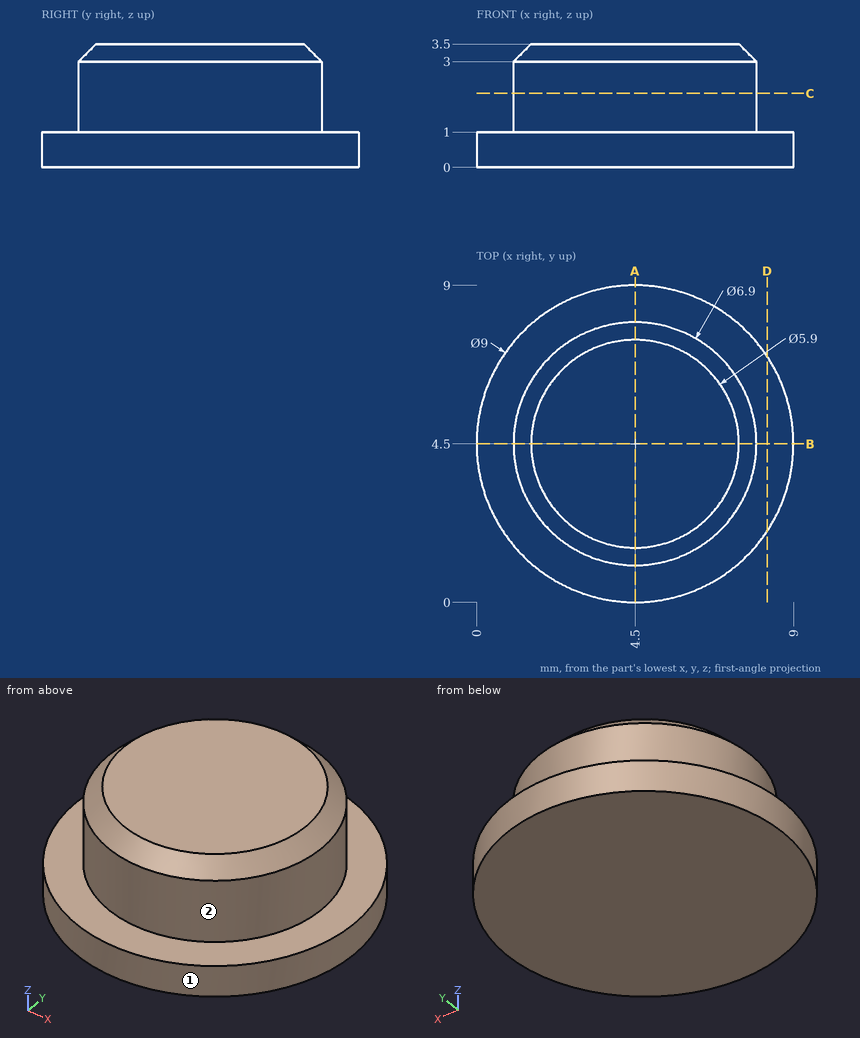
Can you work these out from the drawing? Everything is in mm from the part's minimum corner. A direction names the side the tool comes from. Give positions to 0.01 mm unless a question says otherwise; leave off trailing zeros. Loops run counter-clockwise (first coordinate to the right, second up) from the corner with the lowest first, then second, coordinate; pieces in that order, holes last. Notation, with made-up numbers: (-38.75, -6) -> (1.25, -6) arc R4 cw to (1.25, 0) -> close; hole circle Ø6 at (-8, -12.5). An arc over 180 degrees is marked (long way). Return JSON: item names as keys, results as strings.
Q1. I want a section at C-C, the plane z = 2.1. List the corners of the cut face in (x, y) for me, then the cut area to 3 significant figures.
Checks:
{"outline": "circle Ø6.9 at (4.5, 4.5)", "area": "37.4 mm2"}
Q2. I want a section at D-D, the plane x = 8.25. List the corners of the cut face in (y, z) for me.
Checks:
{"outline": "(2.01, 0) -> (6.99, 0) -> (6.99, 1) -> (2.01, 1) -> close"}
Q3. I need wall thicknesses on probe 1 along Z at (x, y) = (1.75, 7.5); probe 2 along X at (y, z) = (6.25, 0.35); probe 3 along X at (y, z) = (5.75, 0.45). Which ranges of each line are inside material? Lowest first, please.
Checks:
{"probe 1": "z = 0 to 1", "probe 2": "x = 0.35 to 8.65", "probe 3": "x = 0.18 to 8.82"}
Q4. On a 3-axis mill with a long thin cutter (end or side, diameter ignored), from which of +Z, -Z, +X, -X, +Y, -Y can I reach the whole of each face in a straight line? I mean the marked faces 1 and 2. Say none if no direction works.
Checks:
{"face 1": "+Z, -Z", "face 2": "+Z"}
Q5. I want a section at A-A, the plane x = 4.5. List the corners of the cut face in (y, z) for me.
Checks:
{"outline": "(0, 0) -> (9, 0) -> (9, 1) -> (7.95, 1) -> (7.95, 3) -> (7.45, 3.5) -> (1.55, 3.5) -> (1.05, 3) -> (1.05, 1) -> (0, 1) -> close"}
Q6. For pin 1 Ø1.5 at (x, z) = (1.5, 1.5) entering from -Y; pin 2 Ø1.5 at (y, z) = (4, 1.5) entering from +X; pin 3 Ø1.5 at (y, z) = (4, 3) entering from -X; pin 4 Ø1.5 at (y, z) = (1.5, 2.5) entering from -X, each with a flat end and sliding along its axis, tell me the tip position at first contact or that it passes through.
Checks:
{"pin 1": "stops at y = 0.72", "pin 2": "stops at x = 9", "pin 3": "stops at x = 1.05", "pin 4": "stops at x = 1.88"}
